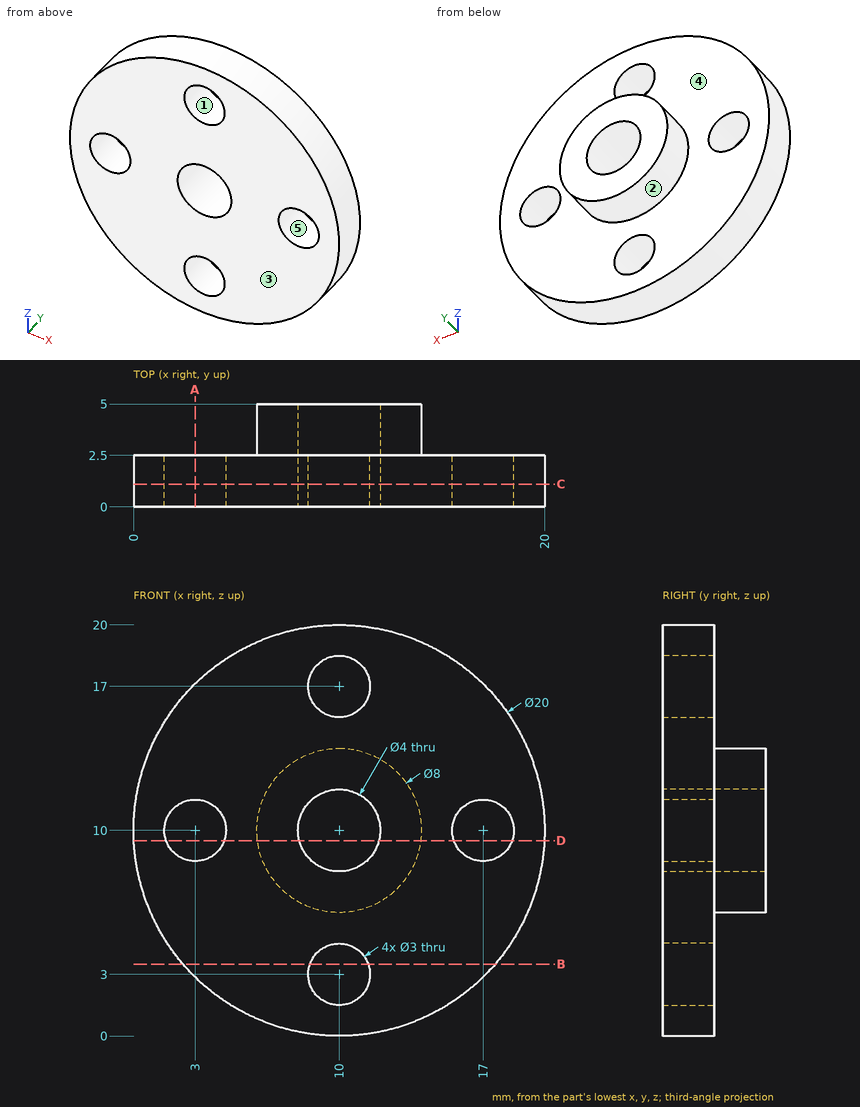
Answer from the drawing. Dimensions are ordinates in mm from the lowest x, y and z of the part. A direction names the side the tool comes from. Give positions to 0.01 mm unless a question says otherwise; leave off trailing zeros. Loops run counter-clockwise (first coordinate to the right, second up) from the corner with the lowest first, then second, coordinate; pieces in that order, holes last.
Item 1: The part is cut by section D-D (z = 9.5). Write down the section's boundary in (x, y).
Item 2: Find the intervals of material crossed by line 1 along X through (y, z) = (1.4, 10); line 2 along X through (y, z) = (3.85, 10); line 3 along Y through (x, z) = (17.5, 3.75), in increasing order.
Item 3: Each of these flat-tipped pins is pushed along its axis until it touches: pin 1 Ø1 at (x, y) = (3.5, 2) entering from +Z; pin 2 Ø1.5 at (y, z) = (4, 17.5) entering from -X; pin 3 Ø4 at (x, z) = (17, 10) entering from +Y; pin 4 Ø3 at (y, z) = (1, 3.5) entering from -X. Where does it stop, or does it pass through?
Item 4: The part is cut by section C-C (y = 1.1). Write down the section's boundary in (x, z).
Item 5: For the marked faces 4 and 5, determine the directions among +Z, -Z, +X, -X, +Y, -Y from which every point of the face is accessible in a straight line to the end or side of a thin tool.
Item 6: The part is cut by section B-B (z = 3.5). Write down the section's boundary in (x, y).
Item 7: The part is cut by section A-A (x = 3). Write down the section's boundary in (y, z), and give its area (3 significant figures).
Item 8: The mould has two halves that part along Z. Classify the marked faces 1, 2 and 3: released by +Z, released by -Z, zero draft, split by the parting line, or undercut.
Taken from the geometry:
1. outline: (0.01, 0) - (1.59, 0) - (1.59, 2.5) - (0.01, 2.5) - close; (4.41, 0) - (8.06, 0) - (8.06, 5) - (6.03, 5) - (6.03, 2.5) - (4.41, 2.5) - close; (11.94, 0) - (15.59, 0) - (15.59, 2.5) - (13.97, 2.5) - (13.97, 5) - (11.94, 5) - close; (18.41, 0) - (19.99, 0) - (19.99, 2.5) - (18.41, 2.5) - close
2. line 1: x = 0 to 1.5, 4.5 to 8, 12 to 15.5, 18.5 to 20
2. line 2: x = 6 to 8, 12 to 14
2. line 3: y = 0 to 2.5
3. pin 1: stops at z = 18
3. pin 2: passes through
3. pin 3: stops at y = 2.5
3. pin 4: stops at x = 1.34
4. outline: circle Ø20 at (10, 10); hole circle Ø3 at (3, 10); hole circle Ø4 at (10, 10); hole circle Ø3 at (10, 3); hole circle Ø3 at (10, 17); hole circle Ø3 at (17, 10)
5. face 4: +Y
5. face 5: +Y, -Y
6. outline: (2.4, 0) - (8.59, 0) - (8.59, 2.5) - (2.4, 2.5) - close; (11.41, 0) - (17.6, 0) - (17.6, 2.5) - (11.41, 2.5) - close
7. outline: (0, 2.86) - (2.5, 2.86) - (2.5, 8.5) - (0, 8.5) - close; (0, 11.5) - (2.5, 11.5) - (2.5, 17.14) - (0, 17.14) - close
7. area: 28.2 mm2
8. face 1: undercut
8. face 2: split by the parting line
8. face 3: zero draft
